Check sheet for the modelled part. Datum: model origin and axes. Units: mm. Face numbers are marked on the shaded views. A direction names the side the tool comes from. Coordinates: 2 decimals unless noted, no trailing zeros. Loops run counter-clockwise (first coordinate to the right, second up) from the corner with the lowest first, then second, coordinate; pieces in that order, holes last. Notation, with made-up numbers: M 63,74 L 86,74 A20 cw 86,84 Z; hole C 26,46.5 d10. An arc over 180 degrees is marked long. Use CSV: the item, a comma, the result in double quotes. Start each with the question number.
(1) Section check C-C on z = -15. Record the cut outline in (x, y).
(2) Section check A-A on y = 0. Record the cut outline in (x, z).
(3) Set-up check for the marked faces 1 and 2: record each of +Z, -Z, +X, -X, +Y, -Y from which the full face is reachable in a straight line by a thin tool's end or side.
(4) Go/stop test with a flat-tipped pin: pin 1 Ø1.5 at (x, z) = (-2, -29.5) entering from +Y. Record where the tip stops, or that it passes through.
(5) Scan lines: line 1 (Z direction, x = 1.25, y = -3.25); line 2 (Z direction, x = 2, y = -0.25); line 3 (X direction, y = -0.5, z = -11). Record each from-to range of solid material in increasing order.
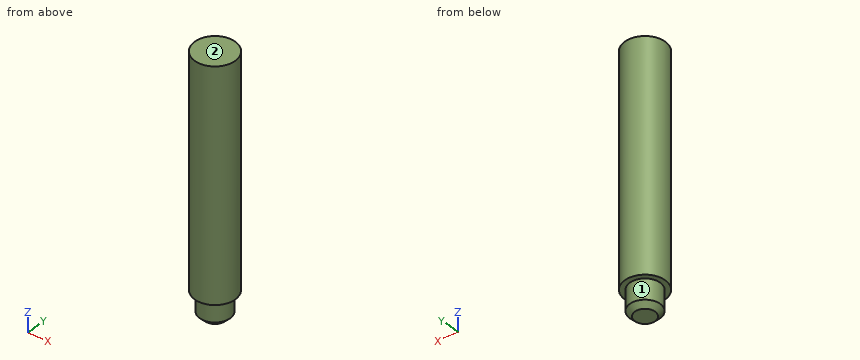
from build123d import *

# Parameters (mm, degrees)
F0_R          = 4
F0_R_2        = 3
F1_DEPTH      = 35
F1_DEPTH_BACK = 10
F2_DEPTH      = 40
F3_SIZE       = 1


with BuildPart() as f1:
    # F0 (on Top) → F1 (new body, two sides)
    with BuildSketch(Plane.XY) as f1_sk:
        Circle(F0_R)
        Circle(F0_R_2, mode=Mode.SUBTRACT)
        Circle(F0_R_2)
    extrude(amount=-F1_DEPTH)
    extrude(f1_sk.sketch, amount=F1_DEPTH_BACK)

    # F0 (on Top) → F2 (join)
    with BuildSketch(Plane.XY):
        Circle(F0_R_2)
    extrude(amount=-F2_DEPTH)

    # F3
    f3_edges = [f1.edges().sort_by_distance(p)[0] for p in [
        (-3, 0, -40),
    ]]
    chamfer(f3_edges, length=F3_SIZE)


solid = f1.part
Outcome:
1,outline,"C 0,0 d8"
2,outline,"M -4,-35 L -3,-35 L -3,-39 L -2,-40 L 2,-40 L 3,-39 L 3,-35 L 4,-35 L 4,10 L -4,10 Z"
3,face 1,"-Z"
3,face 2,"+Z, +X, -X, +Y, -Y"
4,pin 1,"stops at y = 3.8"
5,line 1,"z = -35 to 10"
5,line 2,"z = -39.98 to 10"
5,line 3,"x = -3.97 to 3.97"
